Design review of the part built by this model. Coordinates are the model's own, in mm. A direction names the side the tool comes from. Give positions to 0.01 mm unless a question says otherwise; leave off trailing zeros.
```python
from build123d import *

# Parameters (mm, degrees)
SKETCH2_W           = 406.4
SKETCH2_H           = 6.35
BOSS_EXTRUDE1_DEPTH = 254
SKETCH3_R           = 1.3462
SKETCH3_R_2         = 1.1303
CUT_EXTRUDE1_DEPTH  = 7.35
CUT_EXTRUDE3_DEPTH  = 0.762


with BuildPart() as part:
    # Sketch2 → Boss-Extrude1 (new body)
    with BuildSketch(Plane.XY):
        with Locations((203.2, 3.175)):
            Rectangle(SKETCH2_W, SKETCH2_H)
    extrude(amount=-BOSS_EXTRUDE1_DEPTH)

    # Sketch3 → Cut-Extrude1 (cut, through all)
    with BuildSketch(Plane(origin=(0, 6.35, 0), x_dir=(1, 0, 0), z_dir=(0, 1, 0))):
        with Locations((350.8248, 239.7252)):
            Circle(SKETCH3_R)
        with Locations((373.0752, 239.7252)):
            Circle(SKETCH3_R)
        with Locations((373.0752, 190.5)):
            Circle(SKETCH3_R)
        with Locations((350.8248, 190.5)):
            Circle(SKETCH3_R)
        with Locations((355.9556, 156.9212)):
            Circle(SKETCH3_R_2)
        with Locations((367.9444, 156.9212)):
            Circle(SKETCH3_R_2)
        with Locations((367.9444, 97.0788)):
            Circle(SKETCH3_R_2)
        with Locations((355.9556, 97.0788)):
            Circle(SKETCH3_R_2)
        with Locations((373.0752, 63.5)):
            Circle(SKETCH3_R)
        with Locations((350.8248, 63.5)):
            Circle(SKETCH3_R)
        with Locations((350.8248, 14.2748)):
            Circle(SKETCH3_R)
        with Locations((373.0752, 14.2748)):
            Circle(SKETCH3_R)
    extrude(amount=-CUT_EXTRUDE1_DEPTH, mode=Mode.SUBTRACT)

    # Sketch4 → Cut-Extrude3 (cut)
    with BuildSketch(Plane(origin=(0, 6.35, 0), x_dir=(1, 0, 0), z_dir=(0, 1, 0))):
        with BuildLine():
            Line((346.075, 252.4252), (377.825, 252.4252))
            ThreePointArc((377.825, 252.4252), (379.4125, 250.8377), (377.825, 249.2502))
            Line((377.825, 249.2502), (377.825, 230.2002))
            ThreePointArc((377.825, 230.2002), (379.4125, 228.6127), (377.825, 227.0252))
            Line((377.825, 227.0252), (346.075, 227.0252))
            ThreePointArc((346.075, 227.0252), (344.4875, 228.6127), (346.075, 230.2002))
            Line((346.075, 230.2002), (346.075, 249.2502))
            ThreePointArc((346.075, 249.2502), (344.4875, 250.8377), (346.075, 252.4252))
        make_face()
        with BuildLine():
            Line((346.075, 203.2), (377.825, 203.2))
            ThreePointArc((377.825, 203.2), (379.4125, 201.6125), (377.825, 200.025))
            Line((377.825, 200.025), (377.825, 180.975))
            ThreePointArc((377.825, 180.975), (379.4125, 179.3875), (377.825, 177.8))
            Line((377.825, 177.8), (346.075, 177.8))
            ThreePointArc((346.075, 177.8), (344.4875, 179.3875), (346.075, 180.975))
            Line((346.075, 180.975), (346.075, 200.025))
            ThreePointArc((346.075, 200.025), (344.4875, 201.6125), (346.075, 203.2))
        make_face()
        with BuildLine():
            Line((346.075, 4.7498), (346.075, 23.7998))
            ThreePointArc((346.075, 23.7998), (344.4875, 25.3873), (346.075, 26.9748))
            Line((346.075, 26.9748), (377.825, 26.9748))
            ThreePointArc((377.825, 26.9748), (379.4125, 25.3873), (377.825, 23.7998))
            Line((377.825, 23.7998), (377.825, 4.7498))
            ThreePointArc((377.825, 4.7498), (379.4125, 3.1623), (377.825, 1.5748))
            Line((377.825, 1.5748), (346.075, 1.5748))
            ThreePointArc((346.075, 1.5748), (344.4875, 3.1623), (346.075, 4.7498))
        make_face()
        with BuildLine():
            Line((346.075, 53.975), (346.075, 73.025))
            ThreePointArc((346.075, 73.025), (344.4875, 74.6125), (346.075, 76.2))
            Line((346.075, 76.2), (377.825, 76.2))
            ThreePointArc((377.825, 76.2), (379.4125, 74.6125), (377.825, 73.025))
            Line((377.825, 73.025), (377.825, 53.975))
            ThreePointArc((377.825, 53.975), (379.4125, 52.3875), (377.825, 50.8))
            Line((377.825, 50.8), (346.075, 50.8))
            ThreePointArc((346.075, 50.8), (344.4875, 52.3875), (346.075, 53.975))
        make_face()
    extrude(amount=-CUT_EXTRUDE3_DEPTH, mode=Mode.SUBTRACT)


solid = part.part
```
1. Machinability: for faces 3 (the face through (362, 5.588, -64)), 4 (the face through (200, 0, -125)), which of the approach directions +Z, -Z, +X, -X, +Y, -Y give a long, thin tool a straight path to every point of the face, cutting with its end or side? Answer none if there is none.
Recorded:
face 3: +Y
face 4: +Z, -Z, +X, -X, -Y
2. Draft analysis for pull direction X (two halves, no side actions). For faces 1 (the face through (362, 5.588, -14)), 2 (the face through (200, 6.35, -125)), state which applies: pulls with the +X half, pulls with the -X half, needs draft (parallel to the pull), parting line crosses it, or undercut.
Recorded:
face 1: undercut
face 2: needs draft
3. For pin 1 (2 mm diameter, centred on x = 350.82, z = -63.5, fed in from +Y); pin 2 (7.5 mm diameter, centred on x = 364.5, z = -184.5, fed in from +Y), all flat-tipped, find the tip position at first contact; note any pin that passes through.
Recorded:
pin 1: passes through
pin 2: stops at y = 5.59
